```python
from build123d import *

# Parameters (mm, degrees)
F1_DEPTH = 1981.2
F2_W     = 1739.9
F2_H     = 584.2
F3_DEPTH = 76.2
F4_W     = 158.75
F4_H     = 609.6
F5_DEPTH = 304.8
F6_W     = 1739.9
F6_H     = 1117.6
F7_DEPTH = 76.2


with BuildPart() as f1:
    # F0 (on Front) → F1 (new body)
    with BuildSketch(Plane.XZ):
        Polygon((869.95, -292.1), (869.95, 292.1), (793.75, 292.1), (793.75, -215.9), (-793.75, -215.9), (-793.75, 292.1), (-869.95, 292.1), (-869.95, -292.1), align=None)
    extrude(amount=F1_DEPTH)

    # F2 (on face) → F3 (join)
    with BuildSketch(Plane(origin=(0, 0, 0), x_dir=(-1, 0, 0), z_dir=(0, 1, 0))):
        Rectangle(F2_W, F2_H)
    extrude(amount=F3_DEPTH)

    # F4 (on face) → F5 (join)
    with BuildSketch(Plane.XY.offset(-215.9)):
        with Locations((-714.375, -914.4)):
            Rectangle(F4_W, F4_H)
        with Locations((714.375, -914.4)):
            Rectangle(F4_W, F4_H)
    extrude(amount=F5_DEPTH)

    # F6 (on face) → F7 (join)
    with BuildSketch(Plane(origin=(0, 76.2, 0), x_dir=(-1, 0, 0), z_dir=(0, 1, 0))):
        with Locations((0, 266.7)):
            Rectangle(F6_W, F6_H)
    extrude(amount=F7_DEPTH)


solid = f1.part
```
Geometry: final body of the model. Coordinates: model frame, mm. A direction names the side the tool comes from. Round coordinates to 2 decimals unless told otherwise and drop trailing zeros. Write each loop counter-clockwise with the first axis right and the second up, starting at its lowest first coordinate (ties: lowest second). Pieces come first, ordered by that corner, then holes.
Item 1: Section query B-B (x = 659). Return loops of the section in (y, z), plus the area to 3 significant figures.
Item 2: Material intervals for L1, parallel to X at y = -1450, z = -91; L2, parallel to X at y = -791.5, z = -203.5; L3, parallel to Y at x = -7.5, z = 159, sorted ascending.
Item 3: Section query A-A (z = 177.5). Return loops of the section in (x, y).
Item 4: Set-up query: faces 1 (the face through (-793.75, -977, 91)), 2 (the face through (713, -910, 88.9)), 3 (the face through (4, 33, 292.1)), 4 (the face through (12, -929, -292.1)). Return all of +Z, -Z, +X, -X, +Y, -Y with unobstructed straight access to the full face (end or side cutting, diameter ignored); none if empty.
Item 5: Pin query (flat end, axial travel): P1, Ø6, axis at x = -228, z = 578.5, coming from the -Y side. Return the tip coordinate at first contact, or that it passes through.
Item 6: Section query C-C (y = -937.5). Return loops of the section in (x, z), plus the area to 3 significant figures.
Item 7: Mould query, pull axis X, two halves, no side actions, for faces 5 (the face through (713, -1219.2, -66)), 6 (the face through (-869.95, -929, 11)), 7 (the face through (869.95, -929, 11)), 8 (the face through (12, 76.2, 563)). Classes: +X half, -X half, draft (parallel to the pull), parting line (faces both ways), or undercut.
Item 8: Section query D-D (x = 74.5). Return loops of the section in (y, z), plus the area to 3 significant figures.
Completed:
1. outline: (-1981.2, -292.1) - (152.4, -292.1) - (152.4, 825.5) - (76.2, 825.5) - (76.2, 292.1) - (0, 292.1) - (0, -215.9) - (-609.6, -215.9) - (-609.6, 88.9) - (-1219.2, 88.9) - (-1219.2, -215.9) - (-1981.2, -215.9) - close
1. area: 466,000 mm2
2. L1: x = -869.95 to -793.75, 793.75 to 869.95
2. L2: x = -869.95 to -635, 635 to 869.95
2. L3: y = 0 to 152.4
3. outline: (-869.95, -1981.2) - (-793.75, -1981.2) - (-793.75, 0) - (793.75, 0) - (793.75, -1981.2) - (869.95, -1981.2) - (869.95, 152.4) - (-869.95, 152.4) - close
4. face 1: +Z
4. face 2: +Z, -Y
4. face 3: +Z, +X, -X, -Y
4. face 4: -Z, +X, -X, +Y, -Y
5. P1: stops at y = 76.2
6. outline: (-869.95, -292.1) - (869.95, -292.1) - (869.95, 292.1) - (793.75, 292.1) - (793.75, 88.9) - (635, 88.9) - (635, -215.9) - (-635, -215.9) - (-635, 88.9) - (-793.75, 88.9) - (-793.75, 292.1) - (-869.95, 292.1) - close
6. area: 307,000 mm2
7. face 5: undercut
7. face 6: -X half
7. face 7: +X half
7. face 8: draft
8. outline: (-1981.2, -292.1) - (152.4, -292.1) - (152.4, 825.5) - (76.2, 825.5) - (76.2, 292.1) - (0, 292.1) - (0, -215.9) - (-1981.2, -215.9) - close
8. area: 281,000 mm2
